Read the model definition and answer for the solid it produces. Units are mm, in the model's axes. Face numbers are marked on the shaded views. A direction names the side the tool comes from. Coordinates: 2 decimals unless noted, no trailing zeros. Write each loop counter-clockwise with the first axis right and the second up, starting at its lowest first coordinate (ties: lowest second). Pieces come first, ordered by that corner, then holes.
(1) Section C-C on z = 0 is taken. State how many separate pieces and enclosed holes the cut face has, then the cut area to 3 significant figures.
(2) Section A-A on x = 0 is taken. Write down the section's boundary in (y, z).
(3) Which of the six approach directions +Z, -Z, +X, -X, +Y, -Y give full straight-line access (tool end or side, diameter ignored) to the marked faces 4 and 5?
(4) The mould has two halves that part along Z. Classify the marked faces 1, 2 and 3: +Z half, -Z half, draft (parallel to the pull), parting line (faces both ways), or undercut.
(5) Given pin 1 (8 mm diameter, centred on y = 26, z = 4.5, fed in from -X); pin 2 (3 mm diameter, centred on y = 21, z = -17.5, fed in from +X); pin 3 (5.5 mm diameter, centred on x = -45, z = 0, fed in from -Y); pin 4 (10 mm diameter, centred on y = 28.5, z = -21, fed in from -X), each flat-ended and moving along its own axis, determine where each tip first touches the part or whether it passes through.
(6) Section B-B on y = 26 is taken. Write down the section's boundary in (x, z).
(7) Section D-D on x = -14 is taken. Write down the section's boundary in (y, z), then the cut area to 3 significant figures.
(8) Find the intervals of material crossed by probe 1 along Z at (x, y) = (7.5, 33); probe 2 along X at (y, z) = (0.95, 0); probe 3 along X at (y, z) = (10, -5), in increasing order.
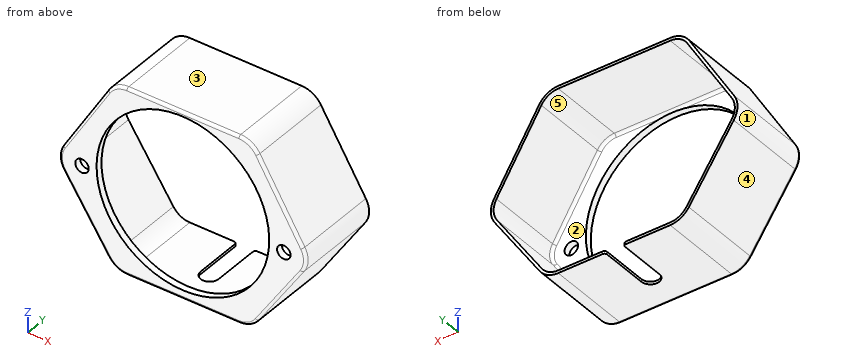
from build123d import *
from build123d.topology import SkipClean

# Parameters (mm, degrees)
ESQUISSE1_R             = 3
BOSS_EXTRU_1_DEPTH      = 3
EXTRU_MINCE1_DEPTH      = 35.3
ENL_V_MAT_EXTRU_1_DEPTH = 10
CONG_1_R                = 1.2


with BuildPart() as part:
    # Esquisse1 → Boss.-Extru.1 (new body)
    with BuildSketch(Plane(origin=(0, 0, 0), x_dir=(1, 0, 0), z_dir=(0, 1, 0))):
        with BuildLine():
            Line((0, 40), (0, 36))
            ThreePointArc((0, 36), (-38.5, -2.5), (0, -41))
            Line((0, -41), (0, -43))
            Line((0, -43), (-24.964670006, -43))
            ThreePointArc((-24.964670006, -43), (-29.868898482, -41.714846129), (-33.512589316, -38.189708611))
            Line((-33.512589316, -38.189708611), (-53.54791931, -5.189708611))
            ThreePointArc((-53.54791931, -5.189708611), (-54.99767043, 0.215837849), (-53.315980127, 5.553780202))
            Line((-53.315980127, 5.553780202), (-33.280650133, 35.553780202))
            ThreePointArc((-33.280650133, 35.553780202), (-29.679656643, 38.818667757), (-24.964670006, 40))
            Line((-24.964670006, 40), (0, 40))
        make_face()
        with Locations(Location((-45, 0, 0), (0, 0, 270))):
            Circle(ESQUISSE1_R, mode=Mode.SUBTRACT)
    extrude(amount=BOSS_EXTRU_1_DEPTH)

    # Esquisse2 → Extru.-Mince1 (add)
    with BuildSketch(Plane(origin=(0, 3, 0), x_dir=(1, 0, 0), z_dir=(0, 1, 0))):
        with BuildLine():
            Line((0, 40), (-24.964670006, 40))
            ThreePointArc((-24.964670006, 40), (-29.679656643, 38.818667757), (-33.280650133, 35.553780202))
            Line((-33.280650133, 35.553780202), (-53.315980127, 5.553780202))
            ThreePointArc((-53.315980127, 5.553780202), (-54.99767043, 0.215837849), (-53.54791931, -5.189708611))
            Line((-53.54791931, -5.189708611), (-33.512589316, -38.189708611))
            ThreePointArc((-33.512589316, -38.189708611), (-29.868898482, -41.714846129), (-24.964670006, -43))
            Line((-24.964670006, -43), (0, -43))
            Line((0, -43), (0, -41.8))
            Line((0, -41.8), (-24.964670006, -41.8))
            ThreePointArc((-24.964670006, -41.8), (-29.280391065, -40.669064594), (-32.486838999, -37.566943577))
            Line((-32.486838999, -37.566943577), (-52.522168993, -4.566943577))
            ThreePointArc((-52.522168993, -4.566943577), (-53.797949978, 0.189937307), (-52.318062511, 4.887326578))
            Line((-52.318062511, 4.887326578), (-32.282732517, 34.887326578))
            ThreePointArc((-32.282732517, 34.887326578), (-29.113858247, 37.760427626), (-24.964670006, 38.8))
            Line((-24.964670006, 38.8), (0, 38.8))
            Line((0, 38.8), (0, 40))
        make_face()
    extrude(amount=EXTRU_MINCE1_DEPTH)

    # Esquisse3 → Enlèv. mat.-Extru.1 (cut)
    with BuildSketch(Plane(origin=(0, 0, -40), x_dir=(-1, 0, 0), z_dir=(0, 0, -1))):
        with BuildLine():
            Line((-4, 16.3), (-4, 38.3))
            ThreePointArc((-4, 38.3), (0, 42.3), (4, 38.3))
            Line((4, 38.3), (4, 16.3))
            ThreePointArc((4, 16.3), (0, 12.3), (-4, 16.3))
        make_face()
    extrude(amount=-ENL_V_MAT_EXTRU_1_DEPTH, mode=Mode.SUBTRACT)

    # Congé1
    cong_1_edges = [part.edges().sort_by_distance(p)[0] for p in [
        (-12.482335003, 3, 41.8),
        (-29.280391065, 3, 40.669064594),
        (-42.504503996, 3, 21.066943577),
        (-53.797949978, 3, -0.189937307),
        (-42.300397514, 3, -19.887326578),
        (-29.113858247, 3, -37.760427626),
        (-12.482335003, 3, -38.8),
        (-4, 38.3, -39.4),
        (-12.482335003, 0, -40),
        (-29.679656643, 0, -38.818667757),
        (-43.29831513, 0, -20.553780202),
        (-54.99767043, 0, -0.215837849),
        (-43.530254313, 0, 21.689708611),
        (-29.868898482, 0, 41.714846129),
        (-12.482335003, 0, 43),
    ]]
    fillet(cong_1_edges, radius=CONG_1_R)

    # Symétrie1: part across plane


with BuildPart() as part_1:
    with SkipClean():  # the faces are left unmerged after this step: merging them gives an invalid solid
        add(part.part)
        add(part.part.mirror(Plane(origin=(0, 3, 41), x_dir=(0, 0, 1), z_dir=(-1, 0, 0))))


solid = part_1.part
Response:
1. separate pieces: 4
1. enclosed holes: 0
1. area: 148 mm2
2. outline: (0, -38.8) arc R1.2 ccw to (1.2, -40) - (12.3, -40) - (12.3, -38.8) - (4.2, -38.8) arc R1.2 cw to (3, -37.6) - (3, -36) - (0, -36) - close; (0, 41) - (3.07, 41) arc R1.2 cw to (4.2, 41.8) - (38.3, 41.8) - (38.3, 43) - (1.2, 43) arc R1.2 ccw to (0, 41.8) - close
3. face 4: -Z, -X, +Y, -Y
3. face 5: +Y
4. face 1: parting line
4. face 2: undercut
4. face 3: +Z half
5. pin 1: stops at x = -54.99
5. pin 2: stops at x = 46.34
5. pin 3: passes through
5. pin 4: stops at x = -46.34
6. outline: (-53.55, 5.19) arc R10 ccw to (-53.32, -5.55) - (-33.28, -35.55) arc R10 ccw to (-24.96, -40) - (-4, -40) - (-4, -38.8) - (-24.96, -38.8) arc R8.8 cw to (-32.28, -34.89) - (-52.32, -4.89) arc R8.8 cw to (-52.52, 4.57) - (-32.49, 37.57) arc R8.8 cw to (-24.96, 41.8) - (24.96, 41.8) arc R8.8 cw to (32.49, 37.57) - (52.52, 4.57) arc R8.8 cw to (52.32, -4.89) - (32.28, -34.89) arc R8.8 cw to (24.96, -38.8) - (4, -38.8) - (4, -40) - (24.96, -40) arc R10 ccw to (33.28, -35.55) - (53.32, -5.55) arc R10 ccw to (53.55, 5.19) - (33.51, 38.19) arc R10 ccw to (24.96, 43) - (-24.96, 43) arc R10 ccw to (-33.51, 38.19) - close
7. outline: (0, -38.8) arc R1.2 ccw to (1.2, -40) - (38.3, -40) - (38.3, -38.8) - (4.2, -38.8) arc R1.2 cw to (3, -37.6) - (3, -33.36) - (0, -33.36) - close; (0, 38.36) - (3, 38.36) - (3, 40.6) arc R1.2 cw to (4.2, 41.8) - (38.3, 41.8) - (38.3, 43) - (1.2, 43) arc R1.2 ccw to (0, 41.8) - close
7. area: 119 mm2
8. probe 1: z = -40 to -38.8, 41.8 to 43
8. probe 2: x = -54.97 to -48, -42 to -38.42, 38.42 to 42, 48 to 54.97
8. probe 3: x = -53.66 to -52.24, 52.24 to 53.66
